The drawing under review shows one solid part. Ordinate dimensions are in mm from its lowest x, y, z. A direction names the side the tool comes from. Coordinates: 2 decimals unless noted, no trailing zeros. Loops run counter-clockwise (first coordinate to the right, second up) from the corner with the lowest first, then second, coordinate; pieces in that order, holes last.
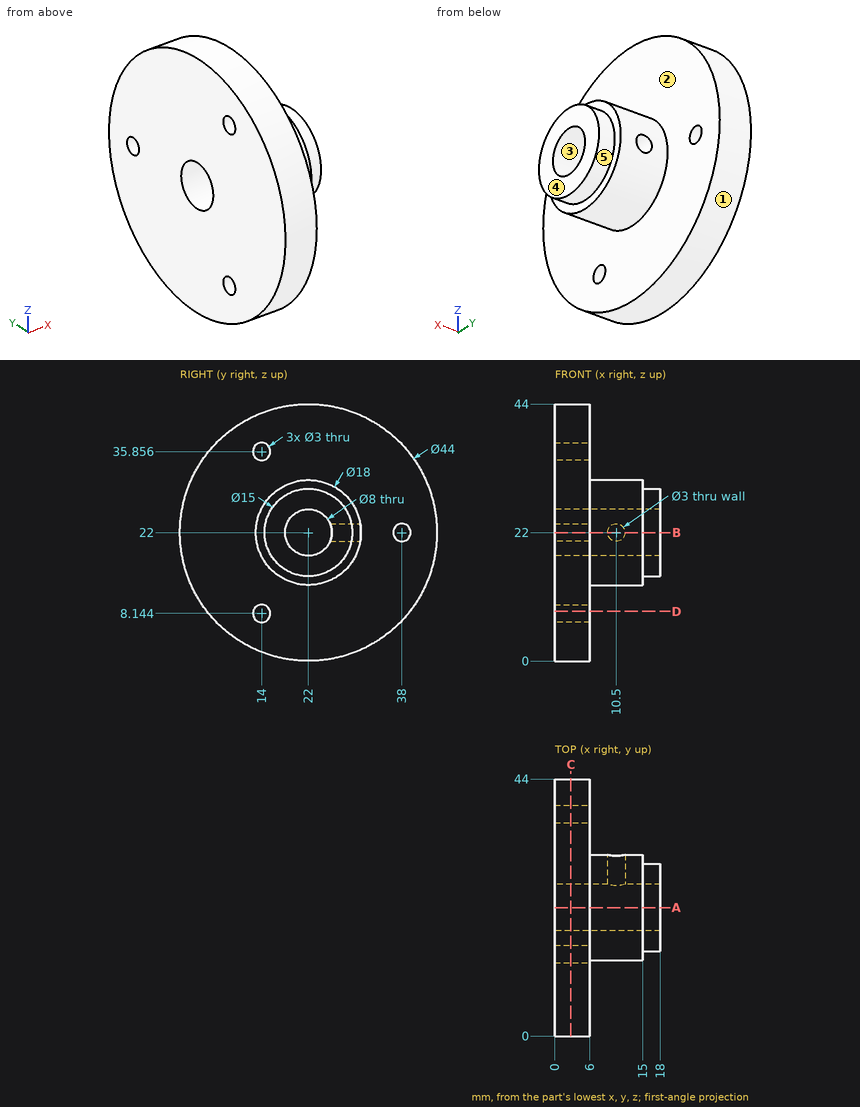
Q1. Take a section at C-C, the plane x = 2.75. Write out the cut boundary in (y, z).
Q2. Machinability: for the marked faces 4 and 5, which of the approach directions +Z, -Z, +X, -X, +Y, -Y give a long, thin tool a straight path to every point of the face, cutting with its end or side? Answer none if there is none.
Q3. Take a section at B-B, the plane z = 22. Write out the cut boundary in (x, y).
Q4. For line 1 (Y direction, x = 3.35, z = 22); line 2 (Z direction, x = 7, y = 22); line 3 (X direction, y = 17, z = 41), list the stretches that pass through material, from the lowest coordinate up.
Q5. Clearance check with flat-ended pins moving along their axes: pin 1 Ø12 at (y, z) = (18, 11.5) entering from +X; pin 2 Ø5 at (y, z) = (22, 22) entering from -X; pin 3 Ø10 at (x, y) = (11.5, 12) entering from +Z; pin 4 Ø1.5 at (y, z) = (21.5, 36) entering from +X. State where each tip first meets the part, or that it passes through.
Q6. Take a section at A-A, the plane y = 22. Write out the cut boundary in (x, z).
Q7. The part is to be moulded in two halves that separate along Y. For the marked faces 1, 2 and 3, say which applies: pulls with the +Y half, pulls with the -Y half, needs draft (parallel to the pull), parting line crosses it, or undercut.
Q8. Take a section at D-D, the plane z = 8.5. Write out the cut boundary in (x, y), then the cut area to 3 significant figures.
Entries:
1. outline: circle Ø44 at (22, 22); hole circle Ø3 at (14, 8.14); hole circle Ø3 at (14, 35.86); hole circle Ø8 at (22, 22); hole circle Ø3 at (38, 22)
2. face 4: +Z, -Z, +X, +Y, -Y
2. face 5: +X
3. outline: (0, 0) - (6, 0) - (6, 13) - (15, 13) - (15, 14.5) - (18, 14.5) - (18, 18) - (0, 18) - close; (0, 26) - (9, 26) - (9, 31) - (6, 31) - (6, 36.5) - (0, 36.5) - close; (0, 39.5) - (6, 39.5) - (6, 44) - (0, 44) - close; (12, 26) - (18, 26) - (18, 29.5) - (15, 29.5) - (15, 31) - (12, 31) - close
4. line 1: y = 0 to 18, 26 to 36.5, 39.5 to 44
4. line 2: z = 13 to 18, 26 to 31
4. line 3: x = 0 to 6
5. pin 1: stops at x = 18
5. pin 2: passes through
5. pin 3: stops at z = 29.48
5. pin 4: stops at x = 6
6. outline: (0, 0) - (6, 0) - (6, 13) - (15, 13) - (15, 14.5) - (18, 14.5) - (18, 18) - (0, 18) - close; (0, 26) - (18, 26) - (18, 29.5) - (15, 29.5) - (15, 31) - (6, 31) - (6, 44) - (0, 44) - close
7. face 1: parting line crosses it
7. face 2: needs draft
7. face 3: undercut
8. outline: (0, 4.63) - (6, 4.63) - (6, 12.54) - (0, 12.54) - close; (0, 15.46) - (6, 15.46) - (6, 39.37) - (0, 39.37) - close
8. area: 191 mm2
